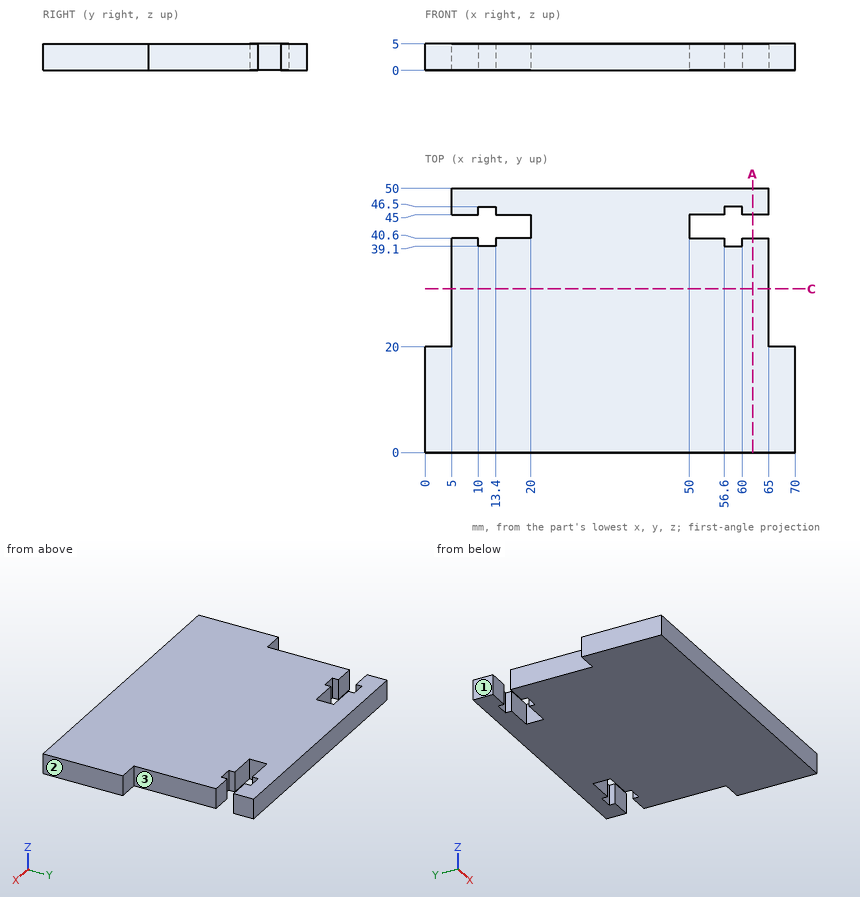
Design review of the part shown in the three views and the two pictorial views. Dimensions are in mm from the part's minimum x, y and z. A direction names the side the tool comes from. Round coordinates to 2 decimals unless told otherwise and drop trailing zeros. Loops run counter-clockwise (first coordinate to the right, second up) from the corner with the lowest first, then second, coordinate; pieces in that order, holes last. Notation, with made-up numbers: (88, -36.5) -> (111, -36.5) arc R20 cw to (111, -13.5) -> close; hole circle Ø7 at (-20, 5.5). An arc over 180 degrees is marked (long way). Answer as CSV lines item,"result".
1) Add section A-A on x = 62. Write out the cut boundary in (y, z).
Geometry results:
outline,"(0, 0) -> (40.6, 0) -> (40.6, 5) -> (0, 5) -> close; (45, 0) -> (50, 0) -> (50, 5) -> (45, 5) -> close"
2) For P1, Ø2, axis at x = 55.5, y = 23.5, coming from the -Z side; P2, Ø1.3, axis at y = 42, z = 1.5, coming from the +X side; P3, Ø1.2, axis at y = 45.5, z = 3, coming from the -X side; P4, Ø0.8, axis at y = 46, z = 3.5, coming from the +X side, all flat-tipped, find the tip position at first contact; note any pin that passes through.
Geometry results:
P1,"stops at z = 0"
P2,"stops at x = 50"
P3,"stops at x = 5"
P4,"stops at x = 65"
3) To check wall thickness, follow line 1 along Y through (x, z) = (18, 0.85); line 2 along X through (y, z) = (46, 3.9); line 3 along X through (y, z) = (44, 0.9). State the ranges of each line that lie inside material, in increasing order. Write a range as from..to.
Geometry results:
line 1,"y = 0..40.6, 45..50"
line 2,"x = 5..10, 13.4..56.6, 60..65"
line 3,"x = 20..50"
4) Add section C-C on y = 31. Write out the cut boundary in (x, z).
Geometry results:
outline,"(5, 0) -> (65, 0) -> (65, 5) -> (5, 5) -> close"
5) Tool access review of the marked faces 1, 2 and 3: name each direction out of +Z, -Z, +X, -X, +Y, -Y from which nothing blocks a thin tool from reaching the whole face with its end or side.
Geometry results:
face 1,"+Z, -Z, -X, +Y"
face 2,"+Z, -Z, +X, +Y, -Y"
face 3,"+Z, -Z, +X, +Y"
